from build123d import *

# Parameters (mm, degrees)
F0_W     = 175.344706
F0_H     = 107.297548
F1_DEPTH = 3.81
F2_R     = 1.27
F3_W     = 73.110506
F3_H     = 41.154918
F4_DEPTH = 2.54
F5_W     = 160.746276
F5_H     = 53.74348
F6_DEPTH = 0.254


with BuildPart() as f1:
    # F0 (on Top) → F1 (new body)
    with BuildSketch(Plane.XY):
        Rectangle(F0_W, F0_H)
    extrude(amount=F1_DEPTH)

    # F2
    f2_edges = [f1.edges().sort_by_distance(p)[0] for p in [
        (87.672353, 0, 0),
        (0, -53.648774, 0),
        (0, 53.648774, 0),
        (-87.672353, 0, 0),
    ]]
    fillet(f2_edges, radius=F2_R)

    # F3 (on face) → F4 (join)
    with BuildSketch(Plane.XY.offset(3.81)):
        with Locations((0, -30.382013)):
            Rectangle(F3_W, F3_H)
    extrude(amount=-F4_DEPTH)

    # F5 (on face) → F6 (join)
    with BuildSketch(Plane.XY.offset(3.81)):
        with Locations((0, 18.277625)):
            Rectangle(F5_W, F5_H)
    extrude(amount=F6_DEPTH)


solid = f1.part
Can you work these out from the model? Positions are in its coordinate system, mm. Give positions to 0.01 mm unless a question says otherwise; leave off trailing zeros. Loops run counter-clockwise (first coordinate to the right, second up) from the corner with the lowest first, then second, coordinate; pieces in that order, holes last. Notation, with made-up numbers: (-31.5, -36) - (25.5, -36) arc R14 cw to (25.5, -22) - close; hole circle Ø1 at (80.5, -30). An arc over 180 degrees is marked (long way). Answer as a JSON object with one key per item and string values.
Q1. Will this pin go through, and if not, where does the flat tip stop? P1, Ø5, axis at x = -17.5, y = -41.5, coming from the +Z side.
Geometry says:
{"P1": "z = 3.81"}
Q2. Imagine slicing it at A-A on x = -47. Write out the boundary of the cut face in (y, z), plus the area to 3 significant figures.
Geometry says:
{"outline": "(-53.65, 1.27) arc R1.27 ccw to (-52.38, 0) - (52.38, 0) arc R1.27 ccw to (53.65, 1.27) - (53.65, 3.81) - (45.15, 3.81) - (45.15, 4.06) - (-8.59, 4.06) - (-8.59, 3.81) - (-53.65, 3.81) - close", "area": "422 mm²"}
Q3. If I drill on L1, parallel to Y at x = -18, z = 3.85; L2, parallel to Z at x = 74.5, y = -11; L3, parallel to Y at x = -27, z = 1.2, over which ranges is the centre line in solid material (lowest first)?
Geometry says:
{"L1": "-8.59 to 45.15", "L2": "0 to 3.81", "L3": "-53.65 to 53.65"}
Q4. Imagine slicing it at B-B on y = -12. Write out the boundary of the cut face in (x, z).
Geometry says:
{"outline": "(-87.67, 1.27) arc R1.27 ccw to (-86.4, 0) - (86.4, 0) arc R1.27 ccw to (87.67, 1.27) - (87.67, 3.81) - (-87.67, 3.81) - close"}
